The listing builds one solid part. Answer for the finished solid, in the listing's coordinates (mm). Face numbers are marked on the shaded views. A direction names the side the tool comes from. Coordinates: 2 decimals unless noted, no trailing zeros. Loops run counter-clockwise (first coordinate to the right, second up) from the corner with the lowest first, then second, coordinate; pieces in that order, holes last. Notation, with made-up numbers: (78.25, 31.25) - (97.25, 31.25) arc R31 cw to (97.25, 70.25) - close; hole circle Ø9 at (6.5, 21). An arc over 180 degrees is marked (long way). Use one line per item in the form item = value. Start each with the question number.
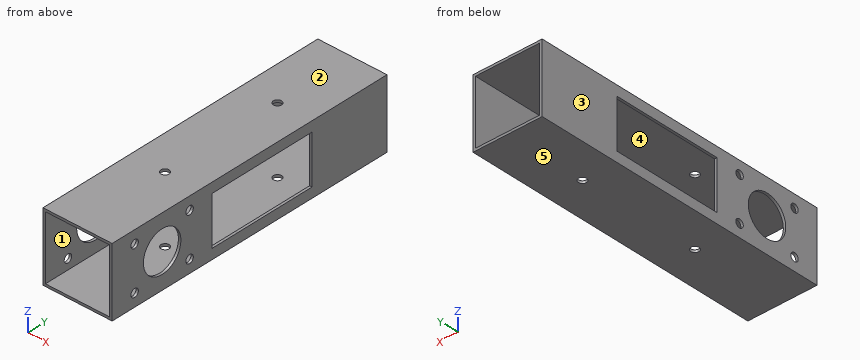
```python
from build123d import *

# Parameters (mm, degrees)
SKETCH1_W           = 25.4
SKETCH1_H           = 25.4
SKETCH1_W_2         = 23.6
SKETCH1_H_2         = 23.6
BOSS_EXTRUDE1_DEPTH = 110
SKETCH2_R           = 7.5
SKETCH2_W           = 18
SKETCH2_H           = 40
CUT_EXTRUDE1_DEPTH  = 25.4
SKETCH3_R           = 1.5
CUT_EXTRUDE2_DEPTH  = 25.4
SKETCH4_R           = 1.5
CUT_EXTRUDE3_DEPTH  = 25.4


with BuildPart() as part:
    # Sketch1 → Boss-Extrude1 (new body)
    with BuildSketch(Plane(origin=(0, 0, 0), x_dir=(1, 0, 0), z_dir=(0, 1, 0))):
        Rectangle(SKETCH1_W, SKETCH1_H)
        Rectangle(SKETCH1_W_2, SKETCH1_H_2, mode=Mode.SUBTRACT)
    extrude(amount=BOSS_EXTRUDE1_DEPTH)

    # Sketch2 → Cut-Extrude1 (cut)
    with BuildSketch(Plane(origin=(12.7, 0, 0), x_dir=(0, 0, -1), z_dir=(1, 0, 0))):
        with Locations((0, 20)):
            Circle(SKETCH2_R)
        with Locations((0, 60)):
            Rectangle(SKETCH2_W, SKETCH2_H)
    extrude(amount=-CUT_EXTRUDE1_DEPTH, mode=Mode.SUBTRACT)

    # Sketch3 → Cut-Extrude2 (cut)
    with BuildSketch(Plane(origin=(0, 0, -12.7), x_dir=(-1, 0, 0), z_dir=(0, 0, -1))):
        with Locations((0, 35)):
            Circle(SKETCH3_R)
        with Locations((0, 80)):
            Circle(SKETCH3_R)
    extrude(amount=-CUT_EXTRUDE2_DEPTH, mode=Mode.SUBTRACT)

    # Sketch4 → Cut-Extrude3 (cut)
    with BuildSketch(Plane(origin=(12.7, 0, 0), x_dir=(0, 0, -1), z_dir=(1, 0, 0))):
        with Locations((8, 9)):
            Circle(SKETCH4_R)
        with Locations(Location((8, 31, 0), (0, 0, 180))):
            Circle(SKETCH4_R)
        with Locations(Location((-8, 9, 0), (0, 0, 180))):
            Circle(SKETCH4_R)
        with Locations((-8, 31)):
            Circle(SKETCH4_R)
    extrude(amount=-CUT_EXTRUDE3_DEPTH, mode=Mode.SUBTRACT)


solid = part.part
```
(1) For the marked faces 1 and 2, determine the directions among +Z, -Z, +X, -X, +Y, -Y from which every point of the face is accessible in a straight line to the end or side of a thin tool.
(2) Find the intervals of material crossed by probe 1 along Y at (x, z) = (0, -12.05); probe 2 along Z at (x, y) = (9.25, 100.5), in increasing order. Write a range as from..to.
(3) A cutting plane is placed at A-A (x = -9). Determine the outline of the cut face in (y, z), then the cut area to 3 significant figures.
(4) A cutting plane is placed at D-D (x = 0). Determine the outline of the cut face in (y, z), then the cut area to 3 significant figures.
(5) A cutting plane is placed at C-C (z = 0). Determine the outline of the cut face in (x, y), then the cut area to 3 significant figures.
(6) Each of these flat-tipped pins is pushed along its axis until it touches: pin 1 Ø10 at (y, z) = (51.5, 2) entering from +X; pin 2 Ø5 at (y, z) = (9, -8) entering from +X. Where does it stop, or does it pass through?
(7) A cutting plane is placed at B-B (y = 74). Determine the outline of the cut face in (x, z), then the cut area to 3 significant figures.
(8) Determine the mould class of the marked faces 3, 4 and 5 for opening direction X: +X half, -X half, draft (parallel to the pull), parting line (faces both ways), or undercut.
Evaluation:
q1.face_1 = +Y, -Y
q1.face_2 = +Z, +X, -X, +Y, -Y
q2.probe_1 = 0..33.5, 36.5..78.5, 81.5..110
q2.probe_2 = -12.7..-11.8, 11.8..12.7
q3.outline = (0, -12.7) - (110, -12.7) - (110, -11.8) - (0, -11.8) - close; (0, 11.8) - (110, 11.8) - (110, 12.7) - (0, 12.7) - close
q3.area = 198 mm^2
q4.outline = (0, -12.7) - (33.5, -12.7) - (33.5, -11.8) - (0, -11.8) - close; (0, 11.8) - (33.5, 11.8) - (33.5, 12.7) - (0, 12.7) - close; (36.5, -12.7) - (78.5, -12.7) - (78.5, -11.8) - (36.5, -11.8) - close; (36.5, 11.8) - (78.5, 11.8) - (78.5, 12.7) - (36.5, 12.7) - close; (81.5, -12.7) - (110, -12.7) - (110, -11.8) - (81.5, -11.8) - close; (81.5, 11.8) - (110, 11.8) - (110, 12.7) - (81.5, 12.7) - close
q4.area = 187 mm^2
q5.outline = (-12.7, 0) - (-11.8, 0) - (-11.8, 12.5) - (-12.7, 12.5) - close; (-12.7, 27.5) - (-11.8, 27.5) - (-11.8, 40) - (-12.7, 40) - close; (-12.7, 80) - (-11.8, 80) - (-11.8, 110) - (-12.7, 110) - close; (11.8, 0) - (12.7, 0) - (12.7, 12.5) - (11.8, 12.5) - close; (11.8, 27.5) - (12.7, 27.5) - (12.7, 40) - (11.8, 40) - close; (11.8, 80) - (12.7, 80) - (12.7, 110) - (11.8, 110) - close
q5.area = 99.0 mm^2
q6.pin_1 = through
q6.pin_2 = 12.7
q7.outline = (-12.7, -12.7) - (12.7, -12.7) - (12.7, -9) - (11.8, -9) - (11.8, -11.8) - (-11.8, -11.8) - (-11.8, -9) - (-12.7, -9) - close; (-12.7, 9) - (-11.8, 9) - (-11.8, 11.8) - (11.8, 11.8) - (11.8, 9) - (12.7, 9) - (12.7, 12.7) - (-12.7, 12.7) - close
q7.area = 55.8 mm^2
q8.face_3 = -X half
q8.face_4 = undercut
q8.face_5 = draft
